Check sheet for the drawn part. Datum: minimum x, y, z corner. Units: mm. A direction names the side the tool comes from. Round coordinates to 2 decimals unless told otherwise and drop trailing zeros. Write each loop counter-clockwise with the first axis right and the second up, starting at its lowest first coordinate (ties: lowest second). Pieces come first, ordered by that corner, then holes. Notation, with made-up numbers: (29, 76.5) - (69, 76.5) arc R13 ccw to (69, 86.5) - close; hole circle Ø8 at (83.5, 77.25). An arc over 180 degrees is marked (long way). Return JSON: item names as keys, results as strings. Group by question number.
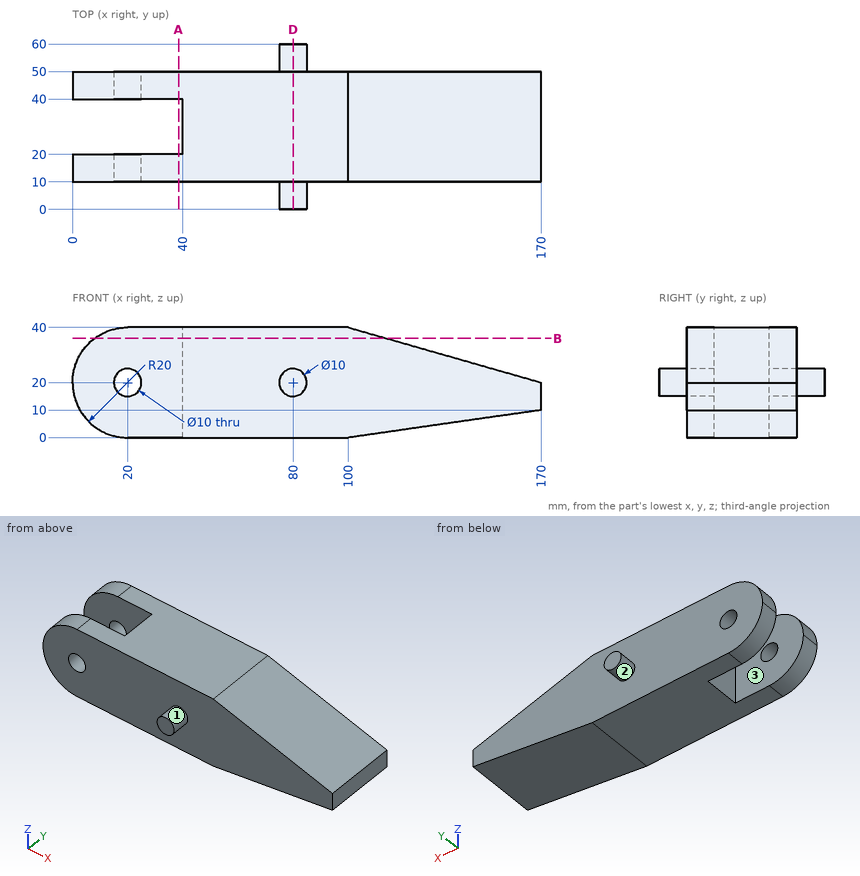
1. Material ranges on line 1 along Y through (x, z) = (14, 25); line 2 along Z through (x, y) = (20, 43); line 3 along Y through (x, z) = (60, 24.5), recorded low to high.
2. Tool access check on the marked faces 1, 2 and 3. Record the directions out of +Z, -Z, +X, -X, +Y, -Y that give a thin tool (end or side, any length) a straight path to the whole face; none if there is none.
3. Section check B-B (z = 36). Enter the section's corners in (x, y).
4. Section check D-D (x = 80). Enter the section's corners in (y, z).
5. Depth check by flat-ended pin: pin 1 Ø12 at (x, z) = (146.5, 22.5) entering from +Y; pin 2 Ø6 at (x, y) = (129, 26.5) entering from +Z; pin 3 Ø3 at (y, z) = (28.5, 26.5) entering from -X. Enter the tip coordinate at first touch or a pass-through.
6. Section check A-A (x = 38.5). Enter the section's corners in (y, z), and give its area (3 significant figures).
Result sheet:
{
 "1": {"line 1": "y = 10 to 20, 40 to 50", "line 2": "z = 0 to 15, 25 to 40", "line 3": "y = 10 to 50"},
 "2": {"face 1": "-Y", "face 2": "+Y", "face 3": "+Z, -Z, -X"},
 "3": {"outline": "(8, 10) - (114, 10) - (114, 50) - (8, 50) - (8, 40) - (40, 40) - (40, 20) - (8, 20) - close"},
 "4": {"outline": "(0, 15) - (10, 15) - (10, 0) - (50, 0) - (50, 15) - (60, 15) - (60, 25) - (50, 25) - (50, 40) - (10, 40) - (10, 25) - (0, 25) - close"},
 "5": {"pin 1": "stops at y = 50", "pin 2": "stops at z = 32.57", "pin 3": "stops at x = 40"},
 "6": {"outline": "(10, 0) - (20, 0) - (20, 40) - (10, 40) - close; (40, 0) - (50, 0) - (50, 40) - (40, 40) - close", "area": "800 mm²"}
}
